from build123d import *

# Parameters (mm, degrees)
SKETCH2_W           = 76.2
SKETCH2_H           = 19.05
BOSS_EXTRUDE1_DEPTH = 215.9
SKETCH3_R           = 3.5
CUT_EXTRUDE1_DEPTH  = 20.05
SKETCH4_R           = 2.5
CUT_EXTRUDE2_DEPTH  = 20.05


with BuildPart() as part:
    # Sketch2 → Boss-Extrude1 (new body)
    with BuildSketch(Plane.XY):
        with Locations((38.1, 9.525)):
            Rectangle(SKETCH2_W, SKETCH2_H)
    extrude(amount=BOSS_EXTRUDE1_DEPTH)

    # Sketch3 → Cut-Extrude1 (cut, through all)
    with BuildSketch(Plane(origin=(0, 19.05, 0), x_dir=(1, 0, 0), z_dir=(0, 1, 0))):
        with Locations((12.7, -7.62)):
            Circle(SKETCH3_R)
        with Locations((63.5, -7.62)):
            Circle(SKETCH3_R)
        with Locations((63.5, -74.295)):
            Circle(SKETCH3_R)
        with Locations((12.7, -74.295)):
            Circle(SKETCH3_R)
    extrude(amount=-CUT_EXTRUDE1_DEPTH, mode=Mode.SUBTRACT)

    # Sketch4 → Cut-Extrude2 (cut, through all)
    with BuildSketch(Plane(origin=(0, 19.05, 0), x_dir=(1, 0, 0), z_dir=(0, 1, 0))):
        with Locations((28.575, -203.2)):
            Circle(SKETCH4_R)
        with Locations((60.325, -203.2)):
            Circle(SKETCH4_R)
        with Locations((60.325, -165.1)):
            Circle(SKETCH4_R)
        with Locations((28.575, -165.1)):
            Circle(SKETCH4_R)
    extrude(amount=-CUT_EXTRUDE2_DEPTH, mode=Mode.SUBTRACT)


solid = part.part
Could you check a few things on this model? Use its own coordinates, in mm. Round coordinates to 2 decimals unless told otherwise and drop trailing zeros. Order: outer loops, then holes, each group sorted by start corner. A loop starts at its lowest first (then second) coordinate and runs counter-clockwise, first axis right, second up. Notation, with made-up numbers: M 4.25,-8 L 23.25,-8 A12 ccw 23.25,6 Z; hole C 66,27 d2. An arc over 180 degrees is marked long. One line per item, written item: value.
(1) Imagine slicing it at A-A (x = 12.7). Write out the boundary of the cut face in (y, z) (3 decimals).
Ans:
outline: M 0,0 L 19.05,0 L 19.05,4.12 L 0,4.12 Z; M 0,11.12 L 19.05,11.12 L 19.05,70.795 L 0,70.795 Z; M 0,77.795 L 19.05,77.795 L 19.05,215.9 L 0,215.9 Z
(2) Imagine slicing it at B-B (z = 203.2). Write out the boundary of the cut face in (x, y) (3 decimals), and give its area (3 significant figures).
Ans:
outline: M 0,0 L 26.075,0 L 26.075,19.05 L 0,19.05 Z; M 31.075,0 L 57.825,0 L 57.825,19.05 L 31.075,19.05 Z; M 62.825,0 L 76.2,0 L 76.2,19.05 L 62.825,19.05 Z
area: 1,260 mm^2
(3) I need wall thicknesses on line 1 along X through (y, z) = (14.25, 7.62); line 2 along X through (y, z) = (4.75, 203.2) (3 decimals); line 3 along Z through (x, y) = (63.5, 4.25) (3 decimals). Which ranges of each line are inside material? Lowest first, please. Write a range as from..to.
Ans:
line 1: x = 0..9.2, 16.2..60, 67..76.2
line 2: x = 0..26.075, 31.075..57.825, 62.825..76.2
line 3: z = 0..4.12, 11.12..70.795, 77.795..215.9
(4) If we mould it in two halves opening along X, with no side actions, what happens to faces 1 (the flat face through (76.2, 9, 106)), 2 (the cylindrical face through (58.482, 9.658, 163.41)), 3 (the flat face through (38, 19.05, 106))? For each: released by +X, released by -X, zero draft, split by the parting line, or undercut.
Ans:
face 1: released by +X
face 2: undercut
face 3: zero draft
